The model under review builds one solid part; all positions refer to its coordinate system, in mm. A direction names the side the tool comes from. Coordinates: 2 decimals unless noted, no trailing zeros. Order: outer loops, then holes, each group sorted by start corner. A loop starts at its lowest first (then second) coordinate and runs counter-clockwise, first axis right, second up. Notation, with made-up numbers: (54, -15) -> (99, -15) arc R14 cw to (99, 6) -> close; hole circle Ø3 at (62, 30.25). An arc over 180 degrees is marked (long way). Use one line per item in the form item = value.
from build123d import *

# Parameters (mm, degrees)
SKETCH_15_W                      = 105
SKETCH_15_H                      = 678
SM_BASE_FLANGE_1_DEPTH           = 0.8
SM_EDGE_FLANGE_1_STRIP_W         = 5.2
SM_EDGE_FLANGE_1_STRIP_H         = 0.8
SM_EDGE_FLANGE_1_STRIP_CUT_DEPTH = 678
SM_EDGE_FLANGE_1_DEPTH           = 678
SM_EDGE_FLANGE_2_STRIP_W         = 5.2
SM_EDGE_FLANGE_2_STRIP_H         = 0.8
SM_EDGE_FLANGE_2_STRIP_CUT_DEPTH = 678
SM_EDGE_FLANGE_2_DEPTH           = 678
SM_EDGE_FLANGE_3_STRIP_W         = 5.2
SM_EDGE_FLANGE_3_STRIP_H         = 0.8
SM_EDGE_FLANGE_3_STRIP_CUT_DEPTH = 678
SM_EDGE_FLANGE_3_DEPTH           = 678
SM_EDGE_FLANGE_4_STRIP_W         = 5.2
SM_EDGE_FLANGE_4_STRIP_H         = 0.8
SM_EDGE_FLANGE_4_STRIP_CUT_DEPTH = 678
SM_EDGE_FLANGE_4_DEPTH           = 678
SKETCH_31_W                      = 16
SKETCH_31_H                      = 14.5
CUT_EXTRUDE_1_DEPTH              = 2
SM_EDGE_FLANGE_5_STRIP_W         = 5.2
SM_EDGE_FLANGE_5_STRIP_H         = 0.8
SM_EDGE_FLANGE_5_STRIP_CUT_DEPTH = 649
SM_EDGE_FLANGE_5_DEPTH           = 649
SKETCH_35_R                      = 1.75
CUT_EXTRUDE_2_DEPTH              = 10
SKETCH_36_R                      = 3
SKETCH_36_R_2                    = 1.25
EXTRUDE_1_DEPTH                  = 3
PATTERN_LINEAR_1_COUNT           = 2
PATTERN_LINEAR_1_PITCH           = 315
PATTERN_LINEAR_1_COUNT_DIR2      = 2
PATTERN_LINEAR_1_PITCH_DIR2      = 315
HOLE_WIZARD_4_0_4_1_D            = 4
HOLE_WIZARD_4_0_4_1_DEPTH        = 5.2
HOLE_WIZARD_4_0_4_1_TIP          = 1.201721238


# Sheet-metal steps are written as plain solids
with BuildPart() as part:
    # 草图15 → 基体-法兰1 (new body)
    with BuildSketch(Plane.XY):
        Rectangle(SKETCH_15_W, SKETCH_15_H)
    extrude(amount=-SM_BASE_FLANGE_1_DEPTH)

    # 边线-法兰1 strip (across the edge) → 边线-法兰1 strip cut (cut)
    with BuildSketch(Plane(origin=(52.5, 339, -0.8), x_dir=(-1, 0, 0), z_dir=(0, -1, 0))):
        with Locations((-0.8, -0.4)):
            Rectangle(SM_EDGE_FLANGE_1_STRIP_W, SM_EDGE_FLANGE_1_STRIP_H)
    extrude(amount=SM_EDGE_FLANGE_1_STRIP_CUT_DEPTH, mode=Mode.SUBTRACT)

    # 边线-法兰1 section (across the edge) → 边线-法兰1 (add)
    with BuildSketch(Plane(origin=(52.5, 339, -0.8), x_dir=(-1, 0, 0), z_dir=(0, -1, 0))):
        with BuildLine():
            Line((0, 1), (0, 24.2))
            Line((0, 24.2), (0.8, 24.2))
            Line((0.8, 24.2), (0.8, 1))
            ThreePointArc((0.8, 1), (1.092893219, 0.292893219), (1.8, 0))
            Line((1.8, 0), (1.8, -0.8))
            ThreePointArc((1.8, -0.8), (0.527207794, -0.272792206), (0, 1))
        make_face()
    extrude(amount=SM_EDGE_FLANGE_1_DEPTH)

    # 边线-法兰2 strip (across the edge) → 边线-法兰2 strip cut (cut)
    with BuildSketch(Plane(origin=(51.7, 339, -25), x_dir=(0, 0, 1), z_dir=(0, -1, 0))):
        with Locations((-0.8, -0.4)):
            Rectangle(SM_EDGE_FLANGE_2_STRIP_W, SM_EDGE_FLANGE_2_STRIP_H)
    extrude(amount=SM_EDGE_FLANGE_2_STRIP_CUT_DEPTH, mode=Mode.SUBTRACT)

    # 边线-法兰2 section (across the edge) → 边线-法兰2 (add)
    with BuildSketch(Plane(origin=(51.7, 339, -25), x_dir=(0, 0, 1), z_dir=(0, -1, 0))):
        with BuildLine():
            Line((0, 1), (0, 9.2))
            Line((0, 9.2), (0.8, 9.2))
            Line((0.8, 9.2), (0.8, 1))
            ThreePointArc((0.8, 1), (1.092893219, 0.292893219), (1.8, 0))
            Line((1.8, 0), (1.8, -0.8))
            ThreePointArc((1.8, -0.8), (0.527207794, -0.272792206), (0, 1))
        make_face()
    extrude(amount=SM_EDGE_FLANGE_2_DEPTH)

    # 边线-法兰3 strip (across the edge) → 边线-法兰3 strip cut (cut)
    with BuildSketch(Plane(origin=(-52.5, -339, -0.8), x_dir=(1, 0, 0), z_dir=(0, 1, 0))):
        with Locations((-0.8, -0.4)):
            Rectangle(SM_EDGE_FLANGE_3_STRIP_W, SM_EDGE_FLANGE_3_STRIP_H)
    extrude(amount=SM_EDGE_FLANGE_3_STRIP_CUT_DEPTH, mode=Mode.SUBTRACT)

    # 边线-法兰3 section (across the edge) → 边线-法兰3 (add)
    with BuildSketch(Plane(origin=(-52.5, -339, -0.8), x_dir=(1, 0, 0), z_dir=(0, 1, 0))):
        with BuildLine():
            Line((0, 1), (0, 14.2))
            Line((0, 14.2), (0.8, 14.2))
            Line((0.8, 14.2), (0.8, 1))
            ThreePointArc((0.8, 1), (1.092893219, 0.292893219), (1.8, 0))
            Line((1.8, 0), (1.8, -0.8))
            ThreePointArc((1.8, -0.8), (0.527207794, -0.272792206), (0, 1))
        make_face()
    extrude(amount=SM_EDGE_FLANGE_3_DEPTH)

    # 边线-法兰4 strip (across the edge) → 边线-法兰4 strip cut (cut)
    with BuildSketch(Plane(origin=(-52.5, 339, -15), x_dir=(0, 0, 1), z_dir=(0, -1, 0))):
        with Locations((-0.8, -0.4)):
            Rectangle(SM_EDGE_FLANGE_4_STRIP_W, SM_EDGE_FLANGE_4_STRIP_H)
    extrude(amount=SM_EDGE_FLANGE_4_STRIP_CUT_DEPTH, mode=Mode.SUBTRACT)

    # 边线-法兰4 section (across the edge) → 边线-法兰4 (add)
    with BuildSketch(Plane(origin=(-52.5, 339, -15), x_dir=(0, 0, 1), z_dir=(0, -1, 0))):
        with BuildLine():
            Line((0, 1), (0, 15.2))
            Line((0, 15.2), (0.8, 15.2))
            Line((0.8, 15.2), (0.8, 1))
            ThreePointArc((0.8, 1), (1.092893219, 0.292893219), (1.8, 0))
            Line((1.8, 0), (1.8, -0.8))
            ThreePointArc((1.8, -0.8), (0.527207794, -0.272792206), (0, 1))
        make_face()
    extrude(amount=SM_EDGE_FLANGE_4_DEPTH)

    # 草图31 → 切除-拉伸1 (cut)
    with BuildSketch(Plane(origin=(0, 0, -15), x_dir=(-1, 0, 0), z_dir=(0, 0, -1))):
        with Locations((59.7, -331.75)):
            Rectangle(SKETCH_31_W, SKETCH_31_H)
    cut_extrude_1 = extrude(amount=-CUT_EXTRUDE_1_DEPTH, mode=Mode.SUBTRACT)

    # 镜向1: 切除-拉伸1 across plane
    add(cut_extrude_1.mirror(Plane.ZX), mode=Mode.SUBTRACT)

    # 边线-法兰5 strip (across the edge) → 边线-法兰5 strip cut (cut)
    with BuildSketch(Plane(origin=(-67.7, -324.5, -15), x_dir=(1, 0, 0), z_dir=(0, 1, 0))):
        with Locations((-0.8, -0.4)):
            Rectangle(SM_EDGE_FLANGE_5_STRIP_W, SM_EDGE_FLANGE_5_STRIP_H)
    extrude(amount=SM_EDGE_FLANGE_5_STRIP_CUT_DEPTH, mode=Mode.SUBTRACT)

    # 边线-法兰5 section (across the edge) → 边线-法兰5 (add)
    with BuildSketch(Plane(origin=(-67.7, -324.5, -15), x_dir=(1, 0, 0), z_dir=(0, 1, 0))):
        with BuildLine():
            Line((0, 1), (0, 5.2))
            Line((0, 5.2), (0.8, 5.2))
            Line((0.8, 5.2), (0.8, 1))
            ThreePointArc((0.8, 1), (1.092893219, 0.292893219), (1.8, 0))
            Line((1.8, 0), (1.8, -0.8))
            ThreePointArc((1.8, -0.8), (0.527207794, -0.272792206), (0, 1))
        make_face()
    extrude(amount=SM_EDGE_FLANGE_5_DEPTH)

    # 草图35 → 切除-拉伸2 (cut)
    with BuildSketch(Plane.XY.offset(-14.2)):
        with Locations((-60, 0)):
            Circle(SKETCH_35_R)
    cut_extrude_2 = extrude(amount=-CUT_EXTRUDE_2_DEPTH, mode=Mode.SUBTRACT)

    # 草图36 → 凸台-拉伸1 (add)
    with BuildSketch(Plane(origin=(0, 0, -15), x_dir=(-1, 0, 0), z_dir=(0, 0, -1))):
        with Locations(Location((60, 0, 0), (0, 0, 180))):
            Circle(SKETCH_36_R)
        with Locations((60, 0)):
            Circle(SKETCH_36_R_2, mode=Mode.SUBTRACT)
    extrude_1 = extrude(amount=EXTRUDE_1_DEPTH)

    # 阵列(线性)1: 切除-拉伸2, Extrude 1 2 × 2
    with Locations(*[Vector(0, -1, 0) * (i * PATTERN_LINEAR_1_PITCH) + Vector(0, 1, 0) * (j * PATTERN_LINEAR_1_PITCH_DIR2) for i in range(PATTERN_LINEAR_1_COUNT) for j in range(PATTERN_LINEAR_1_COUNT_DIR2) if (i, j) != (0, 0)]):
        add(cut_extrude_2, mode=Mode.SUBTRACT)
        add(extrude_1)

    # Ø4.0 (4) 直径孔1
    with Locations(Plane.XY):
        with Locations((-42.5, -271), (-42.5, -321), (27.5, -321), (27.5, -271)):
            Hole(HOLE_WIZARD_4_0_4_1_D / 2, depth=HOLE_WIZARD_4_0_4_1_DEPTH)
            with Locations((0, 0, -(HOLE_WIZARD_4_0_4_1_DEPTH + HOLE_WIZARD_4_0_4_1_TIP / 2))):  # 118° drill point
                Cone(0, HOLE_WIZARD_4_0_4_1_D / 2, HOLE_WIZARD_4_0_4_1_TIP, mode=Mode.SUBTRACT)


solid = part.part
Item 1: We need section B-B (y = 272.5). Write out the cut boundary in (x, z), plus the area to 3 significant figures.
Results found:
outline = (-67.7, -20.2) -> (-66.9, -20.2) -> (-66.9, -16) arc R1 cw to (-65.9, -15) -> (-53.5, -15) arc R1.8 ccw to (-51.7, -13.2) -> (-51.7, -1.8) arc R1 cw to (-50.7, -0.8) -> (50.7, -0.8) arc R1 cw to (51.7, -1.8) -> (51.7, -23.2) arc R1 cw to (50.7, -24.2) -> (42.5, -24.2) -> (42.5, -25) -> (50.7, -25) arc R1.8 ccw to (52.5, -23.2) -> (52.5, -1.8) arc R1.8 ccw to (50.7, 0) -> (-50.7, 0) arc R1.8 ccw to (-52.5, -1.8) -> (-52.5, -13.2) arc R1 cw to (-53.5, -14.2) -> (-65.9, -14.2) arc R1.8 ccw to (-67.7, -16) -> close
area = 136 mm²
Item 2: To check wall thickness, follow L1, parallel to Y at x = -60, z = -15.7; L2, parallel to Y at x = -60, z = -14.7; L3, parallel to Y at x = 27.5, z = -0.15. State the ranges of each line that lie inside material, in increasing order. Write a range as from..to.
Results found:
L1 = -318..-316.25, -313.75..-312, -3..-1.25, 1.25..3, 312..313.75, 316.25..318
L2 = -324.5..-316.75, -313.25..-1.75, 1.75..313.25, 316.75..324.5
L3 = -339..-323, -319..-273, -269..339
Item 3: Tool access review of faces 4 (the face through (51.7, 5, -13)), 5 (the face through (-51.7, -5, -8)), 6 (the face through (-52.5, -5, -7)): name each direction out of +Z, -Z, +X, -X, +Y, -Y from which nothing blocks a thin tool from reaching the whole face with its end or side.
Results found:
face_4 = +Y, -Y
face_5 = -Z, +Y, -Y
face_6 = +Z, -X, +Y, -Y
Item 4: Clearance check with flat-ended pins moving along their axes: pin 1 (6 mm diameter, centred on x = -62.5, y = -94.5, fed in from -Z); pin 2 (0.9 mm diameter, centred on x = -52.5, y = -328, fed in from -Z); pin 3 (3 mm diameter, centred on x = -60, y = 0, fed in from +Z). State where each tip first meets the part, or that it passes through.
Results found:
pin_1 = -15
pin_2 = -13
pin_3 = -15
Item 5: Draft analysis for pull direction Y (two halves, no side actions). For faces 1 (the face through (3.6, 339, -0.4)), 2 (the face through (-60, 5, -15)), 3 (the face through (-60, 5, -14.2)), state which applies: released by +Y, released by -Y, zero draft, split by the parting line, or undercut.
Results found:
face_1 = released by +Y
face_2 = undercut
face_3 = zero draft
Item 6: We need section C-C (x = -31.5). Write out the cut boundary in (y, z), plus the area to 3 significant figures.
Results found:
outline = (-339, -0.8) -> (339, -0.8) -> (339, 0) -> (-339, 0) -> close
area = 542 mm²
Item 7: We need section A-A (z = -6). Write out the cut boundary in (x, y).
Results found:
outline = (-52.5, -339) -> (-51.7, -339) -> (-51.7, 339) -> (-52.5, 339) -> close; (51.7, -339) -> (52.5, -339) -> (52.5, 339) -> (51.7, 339) -> close
